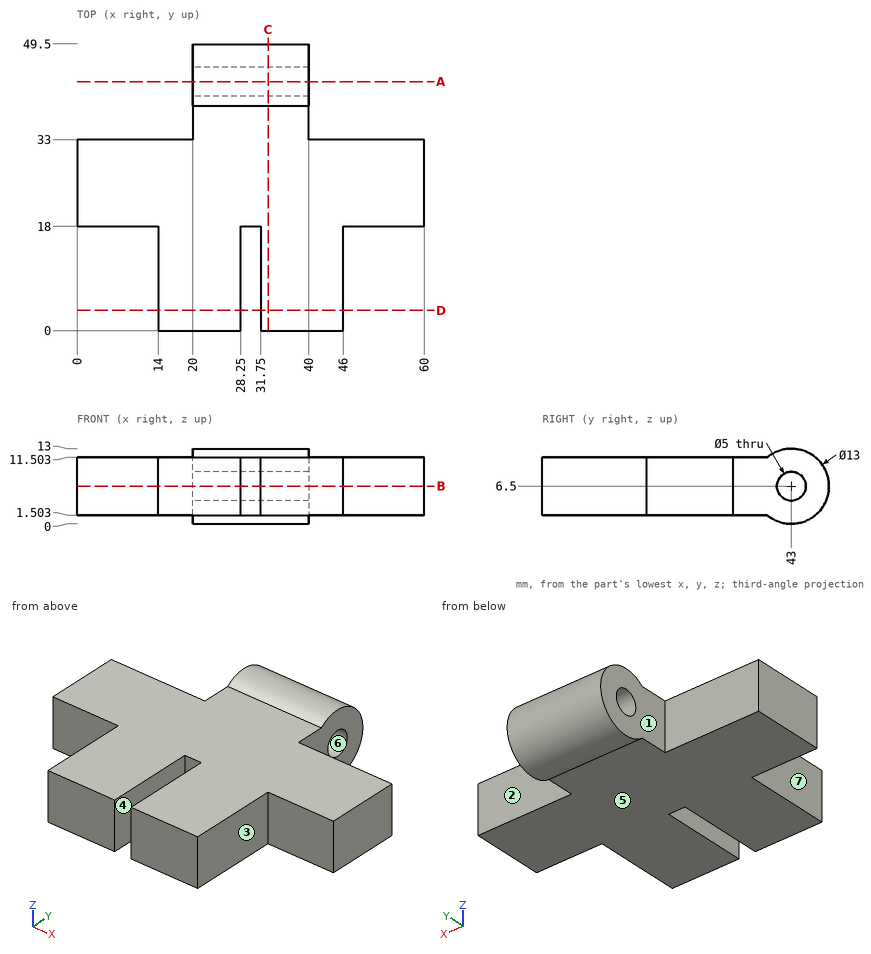
Part print with two shaded views. Sizes in mm from the minimum x, y, z corner. A direction names the side the tool comes from. Round coordinates to 2 decimals unless told otherwise and drop trailing zeros. Order: outer loops, then holes, each group sorted by start corner. A loop starts at its lowest first (then second) coordinate and runs counter-clockwise, first axis right, second up.
(1) Band-saw the part on D-D (y = 3.5). List the corners of the cut face in (x, z), then the cut area to 3 significant figures.
(2) Band-saw the part on A-A (y = 43). List the corners of the cut face in (x, z).
(3) Pin check, flat tips, straight feed: pin 1 (6 mm diameter, centred on y = 37, z = 2.5, fed in from +X); pin 2 (5 mm diameter, centred on y = 13, z = 4.5, fed in from +X); pin 3 (10 mm diameter, centred on x = 33, y = 20.5, fed in from -Z); pin 4 (6 mm diameter, centred on x = 18.5, z = 5, fed in from -Y). Stop position of each tip, or through.
(4) 3-axis set-ups, long thin cutter, end or side, ignore diameter. For the marked faces 1, 2, 3 and 4: which of +Z, -Z, +X, -X, +Y, -Y reach the whole face in a straight line?
(5) Drill centre lines: line 1 (X direction, y = 11.5, z = 10.5); line 2 (Y direction, x = 31, z = 6.5); line 3 (Y direction, x = 33.25, z = 6.5). Where is each one in solid material? Low to high.
(6) Band-saw the part on C-C (x = 33). List the corners of the cut face in (y, z), then the cut area to 3 significant figures.
(7) Band-saw the part on B-B (z = 6.5). List the corners of the cut face in (x, y).
(8) Pull direction Z, two halves, no side cores. Call the marked faces 5, 6 and 7: released by +Z, released by -Z, zero draft, split by the parting line, or undercut.
Verdict:
1. outline: (14, 1.5) - (28.25, 1.5) - (28.25, 11.5) - (14, 11.5) - close; (31.75, 1.5) - (46, 1.5) - (46, 11.5) - (31.75, 11.5) - close
1. area: 285 mm2
2. outline: (20, 0) - (40, 0) - (40, 4) - (20, 4) - close; (20, 9) - (40, 9) - (40, 13) - (20, 13) - close
3. pin 1: stops at x = 40
3. pin 2: stops at x = 46
3. pin 3: stops at z = 1.5
3. pin 4: stops at y = 0
4. face 1: +Z, -Z, -X, +Y
4. face 2: +Z, -Z, +X, +Y
4. face 3: +Z, -Z, +X, -Y
4. face 4: +Z, -Z, -Y
5. line 1: x = 14 to 28.25, 31.75 to 46
5. line 2: y = 18 to 40.5, 45.5 to 49.5
5. line 3: y = 0 to 40.5, 45.5 to 49.5
6. outline: (0, 1.5) - (38.84, 1.5) arc R6.5 ccw (long way) to (38.85, 11.5) - (0, 11.5) - close; hole circle Ø5 at (43, 6.5)
6. area: 485 mm2
7. outline: (0, 18) - (14, 18) - (14, 0) - (28.25, 0) - (28.25, 18) - (31.75, 18) - (31.75, 0) - (46, 0) - (46, 18) - (60, 18) - (60, 33) - (40, 33) - (40, 40.5) - (20, 40.5) - (20, 33) - (0, 33) - close; (20, 45.5) - (40, 45.5) - (40, 49.5) - (20, 49.5) - close
8. face 5: released by -Z
8. face 6: undercut
8. face 7: zero draft
